Here's how the part is built. I have some questions about the finished solid (model axes, mm). Round coordinates to 2 decimals unless told otherwise and drop trailing zeros. Loops run counter-clockwise (first coordinate to the right, second up) from the corner with the lowest first, then second, coordinate; pieces in that order, holes last. Notation, with made-up numbers: M 89,-5.5 L 95,-5.5 A22 ccw 95,6.5 Z; hole C 54,89.5 d7. An arc over 180 degrees is marked long. Write each question's results on one line, items separated by ' | '. Start each with the question number.
```python
from build123d import *

# Parameters (mm, degrees)
F0_R     = 11.2
F1_DEPTH = 5


with BuildPart() as f1:
    # F0 (on Top) → F1 (new body)
    with BuildSketch(Plane.XY):
        with BuildLine():
            Line((28.6, 16.2), (-28.6, 16.2))
            ThreePointArc((-28.6, 16.2), (-39.206602, 11.806602), (-43.6, 1.2))
            Line((-43.6, 1.2), (-43.6, -1.2))
            ThreePointArc((-43.6, -1.2), (-39.206602, -11.806602), (-28.6, -16.2))
            Line((-28.6, -16.2), (28.6, -16.2))
            ThreePointArc((28.6, -16.2), (39.206602, -11.806602), (43.6, -1.2))
            Line((43.6, -1.2), (43.6, 1.2))
            ThreePointArc((43.6, 1.2), (39.206602, 11.806602), (28.6, 16.2))
        make_face()
        with Locations((-27.4, 0)):
            Circle(F0_R, mode=Mode.SUBTRACT)
        Circle(F0_R, mode=Mode.SUBTRACT)
        with Locations((27.4, 0)):
            Circle(F0_R, mode=Mode.SUBTRACT)
    extrude(amount=-F1_DEPTH)


solid = f1.part
```
1. If we mould it in two halves opening along X, with no side actions, what happens to faces 1 (the face through (-38.59, 0.49, -2.46)), 2 (the face through (-39.32, -11.69, -2.46)), 3 (the face through (-10, 7, -5))? For each: released by +X, released by -X, zero draft, split by the parting line, or undercut.
2. I want a section at C-C on z = -1.15. List the corners of the cut face in (x, y) for me, plus the area to 3 significant figures.
3. I need wall thicknesses on line 1 along Y through (x, z) = (-27.4, -3.45); line 2 along X through (y, z) = (-4, -1.4); line 3 along X through (y, z) = (9, -0.3). Which ranges of each line are inside material? Lowest first, please.
4. I want a section at D-D on y = 7. List the corners of the cut face in (x, z) for me, plus the area to 3 significant figures.
5. I want a section at B-B on y = 0. List the corners of the cut face in (x, z) for me, plus the area to 3 significant figures.
6. I want a section at A-A on x = -27.4. List the corners of the cut face in (y, z) for me, plus the area to 3 significant figures.
Outcome:
1) face 1: undercut | face 2: released by -X | face 3: zero draft
2) outline: M -43.6,-1.2 A15 ccw -28.6,-16.2 L 28.6,-16.2 A15 ccw 43.6,-1.2 L 43.6,1.2 A15 ccw 28.6,16.2 L -28.6,16.2 A15 ccw -43.6,1.2 Z; hole C -27.4,0 d22.4; hole C 0,0 d22.4; hole C 27.4,0 d22.4 | area: 1,450 mm2
3) line 1: -16.2 to -11.2, 11.2 to 16.2 | line 2: -43.34 to -37.86, -16.94 to -10.46, 10.46 to 16.94, 37.86 to 43.34 | line 3: -41.41 to -34.07, -20.73 to -6.67, 6.67 to 20.73, 34.07 to 41.41
4) outline: M -42.43,-5 L -36.14,-5 L -36.14,0 L -42.43,0 Z; M -18.66,-5 L -8.74,-5 L -8.74,0 L -18.66,0 Z; M 8.74,-5 L 18.66,-5 L 18.66,0 L 8.74,0 Z; M 36.14,-5 L 42.43,-5 L 42.43,0 L 36.14,0 Z | area: 162 mm2
5) outline: M -43.6,-5 L -38.6,-5 L -38.6,0 L -43.6,0 Z; M -16.2,-5 L -11.2,-5 L -11.2,0 L -16.2,0 Z; M 11.2,-5 L 16.2,-5 L 16.2,0 L 11.2,0 Z; M 38.6,-5 L 43.6,-5 L 43.6,0 L 38.6,0 Z | area: 100 mm2
6) outline: M -16.2,-5 L -11.2,-5 L -11.2,0 L -16.2,0 Z; M 11.2,-5 L 16.2,-5 L 16.2,0 L 11.2,0 Z | area: 50.0 mm2
